Job drawing, mm, ordinate dimensions from the low corner. One solid piece. Round coordinates to 2 decimals unless told otherwise and drop trailing zeros. Order: outer loops, then holes, each group sorted by start corner. A loop starts at its lowest first (then second) coordinate and runs counter-clockwise, first axis right, second up. Notation, with made-up numbers: (88.25, -4.5) - (121.25, -4.5) arc R5 cw to (121.25, 3.5) - close; hole circle Ø1 at (-30.5, -29.75). An arc over 180 degrees is marked (long way). Use one line per item in the form item = value. Start each with the question number.
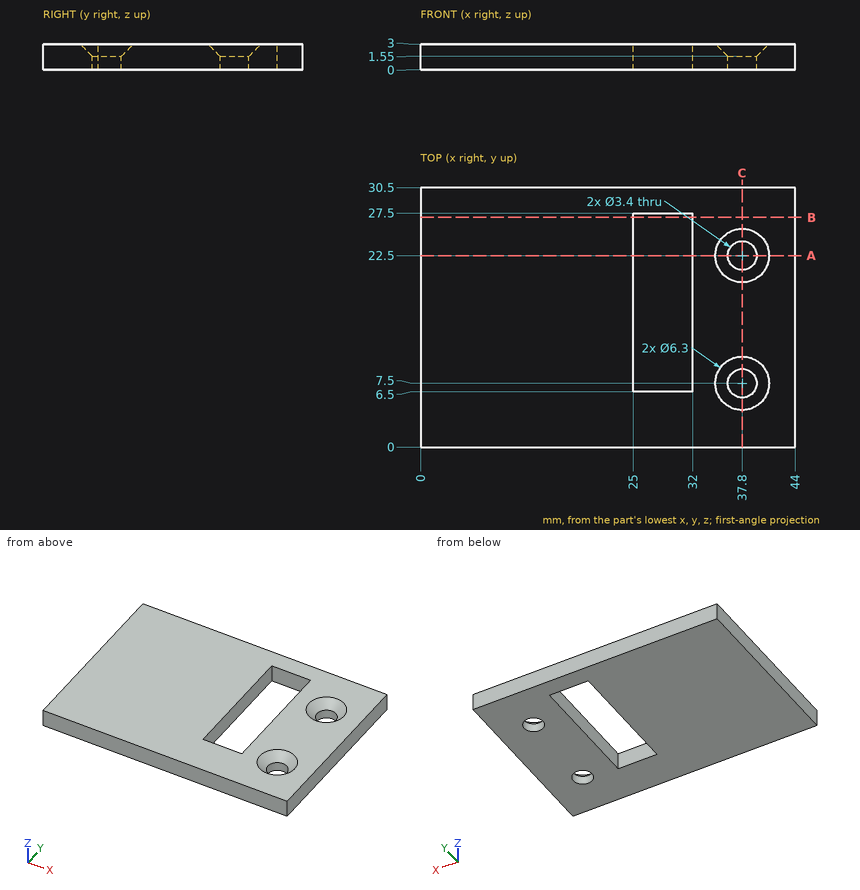
(1) Wall check: line 1 (X direction, y = 22.5, z = 0.7); line 2 (Y direction, x = 37.8, z = 0.75); line 3 (Y direction, x = 25.5, z = 1.35). Give the ranges that are in metal, low to high. Write a range as [from, to].
(2) Flat gauge pin, fed straight in: P1, Ø4.5, axis at x = 37.8, y = 7.5, coming from the +Z side. Where does the tip first touch, or does it go through?
(3) Slice it at B-B (y = 27). Give the cut face in (x, z).
(4) Slice it at A-A (y = 22.5). Give the cut face in (x, z).
(5) Slice it at C-C (x = 37.8). Give the cut face in (y, z), and give its area (3 significant figures).
Results list:
q1.line_1 = [0, 25], [32, 36.1], [39.5, 44]
q1.line_2 = [0, 5.8], [9.2, 20.8], [24.2, 30.5]
q1.line_3 = [0, 6.5], [27.5, 30.5]
q2.P1 = 2.1
q3.outline = (0, 0) - (25, 0) - (25, 3) - (0, 3) - close; (32, 0) - (44, 0) - (44, 3) - (32, 3) - close
q4.outline = (0, 0) - (25, 0) - (25, 3) - (0, 3) - close; (32, 0) - (36.1, 0) - (36.1, 1.55) - (34.65, 3) - (32, 3) - close; (39.5, 0) - (44, 0) - (44, 3) - (40.95, 3) - (39.5, 1.55) - close
q5.outline = (0, 0) - (5.8, 0) - (5.8, 1.55) - (4.35, 3) - (0, 3) - close; (9.2, 0) - (20.8, 0) - (20.8, 1.55) - (19.35, 3) - (10.65, 3) - (9.2, 1.55) - close; (24.2, 0) - (30.5, 0) - (30.5, 3) - (25.65, 3) - (24.2, 1.55) - close
q5.area = 66.9 mm²
